from build123d import *

# Parameters (mm, degrees)
F0_W        = 279.4
F0_H        = 482.6
F1_DEPTH    = 381
F2_R        = 5.08
F3_T1_DEPTH = 401.32
F3_T3_DEPTH = 508
F4_T1_DEPTH = 299.72
F4_T3_DEPTH = 508
F5_T1_DEPTH = 396.24
F6_T        = -2.54


# Not quite as in the source:
# - a fillet or chamfer that OpenCascade refuses, or shapes differently, is made with other operations: its cross-section is extruded or revolved along the edge and cut away or added
# - a shell that OpenCascade refuses in one call is made with other operations: the cavity is built on its own and cut out


with BuildPart() as f1:
    # F0 (on Front) → F1 (new body)
    with BuildSketch(Plane.XZ):
        Rectangle(F0_W, F0_H)
    extrude(amount=F1_DEPTH)

    # F2
    f2_edges = [f1.edges().sort_by_distance(p)[0] for p in [
        (-139.7, -381, 0),
        (0, -381, -241.3),
        (139.7, -381, 0),
        (0, -381, 241.3),
    ]]
    fillet(f2_edges, radius=F2_R)

    # F3: fillet of radius 5.08 on 4 edges, made by hand

    # F3_s2 → F3_t1 (cut)
    with BuildSketch(Plane.XZ.offset(-12.7)):
        with BuildLine():
            ThreePointArc((-139.7, 236.22), (-138.2121024484, 239.8121024484), (-134.62, 241.3))
            Line((-134.62, 241.3), (-139.7, 241.3))
            Line((-139.7, 241.3), (-139.7, 236.22))
        make_face()
        with BuildLine():
            ThreePointArc((-139.7, -236.22), (-138.2121024484, -239.8121024484), (-134.62, -241.3))
            Line((-134.62, -241.3), (-139.7, -241.3))
            Line((-139.7, -241.3), (-139.7, -236.22))
        make_face()
    extrude(amount=F3_T1_DEPTH, mode=Mode.SUBTRACT)

    # F3_s4 → F3_t3 (cut)
    with BuildSketch(Plane.XY.offset(-254)):
        with BuildLine():
            ThreePointArc((-139.7, -5.08), (-138.2121024484, -1.4878975516), (-134.62, 0))
            Line((-134.62, 0), (-139.7, 0))
            Line((-139.7, 0), (-139.7, -5.08))
        make_face()
    extrude(amount=F3_T3_DEPTH, mode=Mode.SUBTRACT)

    # F4: fillet of radius 5.08 on 4 edges, made by hand

    # F4_s2 → F4_t1 (cut)
    with BuildSketch(Plane.YZ.offset(-147.32)):
        with BuildLine():
            ThreePointArc((0, 236.22), (-1.4878975516, 239.8121024484), (-5.08, 241.3))
            Line((-5.08, 241.3), (0, 241.3))
            Line((0, 241.3), (0, 236.22))
        make_face()
        with BuildLine():
            ThreePointArc((0, -236.22), (-1.4878975516, -239.8121024484), (-5.08, -241.3))
            Line((-5.08, -241.3), (0, -241.3))
            Line((0, -241.3), (0, -236.22))
        make_face()
    extrude(amount=F4_T1_DEPTH, mode=Mode.SUBTRACT)

    # F4_s4 → F4_t3 (cut)
    with BuildSketch(Plane.XY.offset(-254)):
        with BuildLine():
            ThreePointArc((134.62, 0), (138.2121024484, -1.4878975516), (139.7, -5.08))
            Line((139.7, -5.08), (139.7, 0))
            Line((139.7, 0), (134.62, 0))
        make_face()
    extrude(amount=F4_T3_DEPTH, mode=Mode.SUBTRACT)

    # F5: fillet of radius 5.08 on 4 edges, made by hand

    # F5_s2 → F5_t1 (cut)
    with BuildSketch(Plane.XZ.offset(-7.62)):
        with BuildLine():
            ThreePointArc((134.62, 241.3), (138.2121024484, 239.8121024484), (139.7, 236.22))
            Line((139.7, 236.22), (139.7, 241.3))
            Line((139.7, 241.3), (134.62, 241.3))
        make_face()
        with BuildLine():
            ThreePointArc((134.62, -241.3), (138.2121024484, -239.8121024484), (139.7, -236.22))
            Line((139.7, -236.22), (139.7, -241.3))
            Line((139.7, -241.3), (134.62, -241.3))
        make_face()
    extrude(amount=F5_T1_DEPTH, mode=Mode.SUBTRACT)

    # F6: a shell. OpenCascade refuses it in one call, so the cavity is built on its own and cut out:
    # the body offset inwards by the wall thickness, plus a prism from it out through each open face.
    f6_core = offset(f1.part, amount=F6_T, mode=Mode.PRIVATE)
    f6_exits = [f6_core.faces().sort_by_distance(p)[0] for p in [
        (0, -378.46, 0),
    ]]
    add(f6_core, mode=Mode.SUBTRACT)
    extrude(f6_exits, amount=-F6_T, mode=Mode.SUBTRACT)


solid = f1.part
Here's how the part is built. I have some questions about the finished solid (model axes, mm). A direction names the side the tool comes from. Coordinates: 2 decimals unless noted, no trailing zeros. Write each loop counter-clockwise with the first axis right and the second up, starting at its lowest first coordinate (ties: lowest second). Pieces come first, ordered by that corner, then holes. Notation, with made-up numbers: (19.5, -24) - (66.5, -24) arc R7 ccw to (66.5, -18) - close; hole circle Ø6 at (-23.5, 49). An arc over 180 degrees is marked (long way). Use one line per item in the form item = value.
1) Suppose I cut it at C-C, the plane x = 38. Write out the boundary of the cut face in (y, z), plus the area to 3 significant figures.
Solved:
outline = (-381, -236.22) arc R5.08 ccw to (-375.92, -241.3) - (-5.08, -241.3) arc R5.08 ccw to (0, -236.22) - (0, 236.22) arc R5.08 ccw to (-5.08, 241.3) - (-375.92, 241.3) arc R5.08 ccw to (-381, 236.22) - (-378.46, 236.22) arc R2.54 cw to (-375.92, 238.76) - (-5.08, 238.76) arc R2.54 cw to (-2.54, 236.22) - (-2.54, -236.22) arc R2.54 cw to (-5.08, -238.76) - (-375.92, -238.76) arc R2.54 cw to (-378.46, -236.22) - close
area = 3,140 mm2
2) I'm going to push flat-ended pins straight in: P1, Ø2, axis at x = -52.5, y = -380, coming from the +Z side; P2, Ø1.3, axis at x = 61.5, y = -379.5, coming from the -Z side; P3, Ø4, axis at x = 16.5, z = -51.5, coming from the -Y side; P4, Ø2, axis at x = -9, z = -131.5, coming from the +Y side. Where does each tip first touch, or does it pass through?
Solved:
P1 = 240.26
P2 = -240.37
P3 = -2.54
P4 = 0
3) Suppose I cut it at A-A, the plane y = -200. Write out the boundary of the cut face in (x, z), plus the area to 3 significant figures.
Solved:
outline = (-139.7, -236.22) arc R5.08 ccw to (-134.62, -241.3) - (134.62, -241.3) arc R5.08 ccw to (139.7, -236.22) - (139.7, 236.22) arc R5.08 ccw to (134.62, 241.3) - (-134.62, 241.3) arc R5.08 ccw to (-139.7, 236.22) - close; hole (-137.16, -236.22) arc R2.54 ccw to (-134.62, -238.76) - (134.62, -238.76) arc R2.54 ccw to (137.16, -236.22) - (137.16, 236.22) arc R2.54 ccw to (134.62, 238.76) - (-134.62, 238.76) arc R2.54 ccw to (-137.16, 236.22) - close
area = 3,830 mm2
4) Thinking about a two-plate mould opening in Y: for faces 3 (the flat face through (-2, -188, 238.76)), 4 (the flat face through (-137.16, -188, -3)), 5 (the flat face through (-2, -2.54, 3)), 6 (the flat face through (-2, -188, -241.3)), which applies, released by +Y, released by -Y, zero draft, split by the parting line, or undercut?
Solved:
face_3 = undercut
face_4 = undercut
face_5 = released by -Y
face_6 = zero draft
5) On a 3-axis mill with a long thin cutter (end or side, diameter ignored), from which of +Z, -Z, +X, -X, +Y, -Y can I reach the whole of each face in a straight line? I mean faces 1 (the flat face through (137.16, -188, -3)), 2 (the flat face through (-2, -188, 241.3)). Say none if no direction works.
Solved:
face_1 = none
face_2 = +Z, +X, -X, +Y, -Y
6) I need wall thicknesses on line 1 (Z direction, x = -60, y = -267.5); line 2 (X direction, y = -243, z = 74); line 3 (Y direction, x = 111, z = -82.5). Which ranges of each line are inside material? Lowest first, please.
Solved:
line_1 = -241.3 to -238.76, 238.76 to 241.3
line_2 = -139.7 to -137.16, 137.16 to 139.7
line_3 = -2.54 to 0
7) Suppose I cut it at B-B, the plane z = -149. Write out the boundary of the cut face in (x, y).
Solved:
outline = (-139.7, -375.92) arc R5.08 ccw to (-134.62, -381) - (-134.62, -378.46) arc R2.54 cw to (-137.16, -375.92) - (-137.16, -5.08) arc R2.54 cw to (-134.62, -2.54) - (134.62, -2.54) arc R2.54 cw to (137.16, -5.08) - (137.16, -375.92) arc R2.54 cw to (134.62, -378.46) - (134.62, -381) arc R5.08 ccw to (139.7, -375.92) - (139.7, -5.08) arc R5.08 ccw to (134.62, 0) - (-134.62, 0) arc R5.08 ccw to (-139.7, -5.08) - close
